Input: part model. Units: mm. Frame: model coordinates. A direction names the side the tool comes from. Coordinates: 2 decimals unless noted, no trailing zeros. Order: outer loops, then holes, each group sorted by start corner. A loop starts at its lowest first (then second) coordinate and runs counter-clockwise, first axis right, second up. Notation, with made-up numbers: (-10.75, 35) -> (-3.75, 35) arc R21 ccw to (-3.75, 43) -> close; hole circle Ø5 at (-38, 6.5). An arc over 180 degrees is marked (long way). Answer as CSV lines item,"result".
from build123d import *

# Parameters (mm, degrees)
SKETCH1_W           = 44
SKETCH1_H           = 42.9
BOSS_EXTRUDE1_DEPTH = 31.8
SKETCH2_OUTSIDE_W   = 59.838
SKETCH2_OUTSIDE_H   = 58.738
CUT_EXTRUDE1_DEPTH  = 31.8
SKETCH6_R           = 5
BOSS_EXTRUDE2_DEPTH = 31.8
BOSS_EXTRUDE3_DEPTH = 0.01


with BuildPart() as part:
    # Sketch1 → Boss-Extrude1 (new body)
    with BuildSketch(Plane(origin=(0, 0, 0), x_dir=(1, 0, 0), z_dir=(0, 1, 0))):
        Rectangle(SKETCH1_W, SKETCH1_H)
    extrude(amount=BOSS_EXTRUDE1_DEPTH)

    # Sketch2 outside → Cut-Extrude1 (cut)
    with BuildSketch(Plane(origin=(0, 31.8, 0), x_dir=(1, 0, 0), z_dir=(0, 1, 0))):
        Rectangle(SKETCH2_OUTSIDE_W, SKETCH2_OUTSIDE_H)
        Polygon((-22, 21.45), (-19, -21.45), (19, -21.45), (22, 21.45), align=None, mode=Mode.SUBTRACT)
    extrude(amount=-CUT_EXTRUDE1_DEPTH, mode=Mode.SUBTRACT)

    # Sketch6 → Boss-Extrude2 (add)
    with BuildSketch(Plane(origin=(0, 0, -21.45), x_dir=(-1, 0, 0), z_dir=(0, 0, -1))):
        with Locations((0.467474435, 15.619515339)):
            Circle(SKETCH6_R)
    extrude(amount=BOSS_EXTRUDE2_DEPTH)

    # Sketch7 → Boss-Extrude3 (add)
    with BuildSketch(Plane.XY.offset(21.45)):
        with BuildLine():
            Line((5.634249571, 3.078676804), (-5.634249571, 3.078676804))
            ThreePointArc((-5.634249571, 3.078676804), (-18.221835549, 15.666262783), (-5.634249571, 28.253848761))
            Line((-5.634249571, 28.253848761), (5.634249571, 28.253848761))
            ThreePointArc((5.634249571, 28.253848761), (18.221835549, 15.666262783), (5.634249571, 3.078676804))
        make_face()
    extrude(amount=BOSS_EXTRUDE3_DEPTH)


solid = part.part
1. Contact query for flat-ended pins moving along their axis: pin 1 (12 mm diameter, centred on x = 11, z = 3, fed in from -Y); pin 2 (8 mm diameter, centred on x = -7, z = -34, fed in from -Y); pin 3 (3 mm diameter, centred on y = 25, z = -8, fed in from +X); pin 4 (1.5 mm diameter, centred on y = 12.5, z = -38.5, fed in from -X). Output: stop coordinate, or through.
Findings:
pin 1,"stops at y = 0"
pin 2,"stops at y = 11.31"
pin 3,"stops at x = 21.16"
pin 4,"stops at x = -4.87"
2. Cut plane C-C (z = -22.5). Return the cut outline in (x, y), plus the area to 3 significant figures.
Findings:
outline,"circle Ø10 at (-0.47, 15.62)"
area,"78.5 mm2"
3. Ray query, line 1 along Z through (x, y) = (-18.5, 5); line 2 along Z through (x, y) = (-8.5, 24.5); line 3 along Y through (x, z) = (-4.5, -38.5). Return the intervals inside material, ascending.
Findings:
line 1,"z = -21.45 to 21.45"
line 2,"z = -21.45 to 21.46"
line 3,"y = 12.66 to 18.58"
4. Reachability of faces 1 (the face through (0.183, 20.577, -37.127)), 2 (the face through (20.48, 16.12, 0.3)) from +Z, -Z, +X, -X, +Y, -Y: full face, straight path, thin tool, end or side. Return the list, or none.
Findings:
face 1,"-Z"
face 2,"+Z, +X, +Y, -Y"
